The listing builds one solid part. Answer for the finished solid, in the listing's coordinates (mm). A direction names the side the tool comes from. Round coordinates to 2 decimals unless told otherwise and drop trailing zeros. Order: outer loops, then holes, each group sorted by start corner. A loop starts at its lowest first (then second) coordinate and runs counter-clockwise, first axis right, second up. Notation, with made-up numbers: (86.5, 51.25) - (138.5, 51.25) arc R13 cw to (138.5, 73.25) - close; hole circle Ø8 at (83.25, 27). An arc over 180 degrees is marked (long way). One line per item, written item: value. Start each with the question number.
1. Section A-A, the plane z = 5.75 is taken. Give the vertices of the cut face in (x, y), then the cut area to 3 significant figures.
2. Section D-D, the plane z = 9.75 is taken. Give the vertices of the cut face in (x, y), then the cut area to 3 significant figures.
3. Flat-ended cylindrical pins translate along their axes: P1, Ø6.5, axis at y = 41, z = 5, coming from the +X side; P2, Ø2, axis at x = 53, z = 3, coming from the +Y side; P3, Ø1.7, axis at x = 5.02, y = 31.5, coming from the +Z side; P4, Ø3.5, axis at x = 50.5, y = 46, coming from the -Z side. Find the tip coordinate at first contact, or state that the pin passes through.
4. For a pull along X with two mould halves and no side action, classify faces 1 (the flat face through (21, 36, 6)), 2 (the flat face through (0, 18, 6)), 3 (the flat face through (21.335, 18, 5)) as released by +X, released by -X, zero draft, split by the parting line, or undercut.
5. Section C-C, the plane y = 6.5 is taken. Give the vertices of the cut face in (x, z).
6. A tool of negligible diameter and unlimited length cuts with its end or side. For faces 4 (the flat face through (44, 21, 1)), 5 (the flat face through (43, 44, 7)), 6 (the flat face through (51, 44, 9)), 7 (the flat face through (33.7, 18, 5)), from which of +Z, -Z, +X, -X, +Y, -Y can it reach the whole face along a straight path? Write none if from no direction.
7. Straight lines are drawn through the part: line 1 (X direction, y = 21, z = 7); line 2 (X direction, y = 7, z = 10.75); line 3 (Z direction, x = 30, y = 21). For each, find the intervals that lie inside material, in ascending order.
8. Section B-B, the plane y = 39.3 is taken. Give the vertices of the cut face in (x, z).
Autodesk Inventor part; units mm, degrees
ref_plane "Work Plane2" through (38.0184, 32.2776, 9) normal (0, 0, 1) x (1, 0, 0)
ref_plane "YZ Plane" through (0, 0, 0) normal (1, 0, 0) x (0, 1, 0)
ref_plane "XZ Plane" through (0, 0, 0) normal (0, 1, 0) x (-1, 0, 0)
ref_plane "Work Plane1" through (22.0339, 196.5, 8) normal (0, 0, 1) x (1, 0, 0)
sketch "Sketch1" plane through (22.0339, 196.5, 8) normal (0, 0, 1) x (1, 0, 0)
  circle A0 centre (5.4838, -190) radius 1.4
  circle A1 centre (27.9838, -190) radius 1.4
  circle A2 centre (-17.0162, -190) radius 1.4
  line L0 (-22.0339, -196.5) -> (32.9661, -196.5)
  line L1 (32.9661, -196.5) -> (32.9661, -186.5)
  line L2 (-22.0339, -186.5) -> (32.9661, -186.5)
  line L3 (-22.0339, -196.5) -> (-22.0339, -186.5)
  circle A3 centre (27.9838, -165) radius 1.4
  circle A4 centre (-17.0162, -165) radius 1.4
  circle A5 centre (5.4838, -165) radius 1.4
  line L4 (32.9661, -160.5) -> (32.9661, -169.5)
  line L5 (-22.0339, -160.5) -> (32.9661, -160.5)
  line L6 (-22.0339, -160.5) -> (-22.0339, -169.5)
  line L7 (32.9661, -169.5) -> (-22.0339, -169.5)
  line L8 (32.9661, -196.5) -> (-22.0339, -196.5)
  line L9 (-22.0339, -196.5) -> (-22.0339, -160.5)
  line L10 (-22.0339, -160.5) -> (32.9661, -160.5)
  line L11 (32.9661, -160.5) -> (32.9661, -196.5)
extrude "Extrusion1" add sketch "Sketch1" along normal blind 4
sketch "Sketch2" plane through (22.0339, 196.5, 8) normal (0, 0, -1) x (-1, 0, 0)
  circle A0 centre (17.0162, -190) radius 1.4
  circle A1 centre (-27.9838, -190) radius 1.4
  circle A2 centre (-5.4838, -190) radius 1.4
  circle A3 centre (-5.4838, -165) radius 1.4
  circle A4 centre (17.0162, -165) radius 1.4
  circle A5 centre (-27.9838, -165) radius 1.4
  line L0 (-32.9661, -196.5) -> (-32.9661, -160.5)
  line L1 (22.0339, -196.5) -> (-32.9661, -196.5)
  line L2 (22.0339, -160.5) -> (22.0339, -196.5)
  line L3 (-32.9661, -160.5) -> (22.0339, -160.5)
  line L4 (22.0339, -196.5) -> (-32.9661, -196.5)
  line L5 (22.0339, -160.5) -> (0.6985, -160.5)
  line L6 (0.6985, -160.5) -> (0.6985, -196.5)
  line L7 (0.6985, -196.5) -> (22.0339, -196.5)
  line L8 (22.0339, -196.5) -> (22.0339, -160.5)
  line L9 (-32.9661, -196.5) -> (-32.9661, -160.5)
  line L10 (-32.9661, -160.5) -> (-11.6661, -160.5)
  line L11 (-11.6661, -160.5) -> (-11.6661, -196.5)
  line L12 (-11.6661, -196.5) -> (-32.9661, -196.5)
  line L13 (-32.9661, -196.5) -> (-32.9661, -160.5)
  line L14 (-11.4661, 0) -> (-11.4661, -200)
  line L15 (0.4985, 0) -> (0.4985, -200)
  dimension "d6" = 0.2
  dimension "d7" = 0.2
extrude "Extrusion2" add sketch "Sketch2" along normal blind 7 contours L0 L3 L11 L1 | L6 L3 L2 L1
sketch "Sketch3" plane through (22.0339, 196.5, 12) normal (0, 0, 1) x (1, 0, 0)
  circle A0 centre (-17.0162, -190) radius 1.4
  circle A1 centre (27.9838, -190) radius 1.4
  circle A2 centre (5.4838, -190) radius 1.4
  circle A3 centre (5.4838, -165) radius 1.4
  circle A4 centre (-17.0162, -165) radius 1.4
  circle A5 centre (27.9838, -165) radius 1.4
  line L0 (32.9661, -196.5) -> (32.9661, -160.5)
  line L1 (32.9661, -160.5) -> (-22.0339, -160.5)
  line L2 (-22.0339, -160.5) -> (-22.0339, -196.5)
  line L3 (-22.0339, -196.5) -> (32.9661, -196.5)
  circle A6 centre (28.987, -157.2) radius 1
  circle A7 centre (28.987, -157.2) radius 1
  circle A8 centre (50.837, -147.5) radius 1
  line L4 (53.837, -158.2) -> (53.837, -154.2581)
  line L5 (53.837, -154.2581) -> (61.5817, -154.2581)
  line L6 (61.5817, -154.2581) -> (61.5817, -153.1829)
  line L7 (61.5817, -153.1829) -> (53.837, -153.1829)
  line L8 (53.837, -153.1829) -> (53.837, -149.448)
  line L9 (53.837, -149.448) -> (61.5817, -149.448)
  line L10 (61.5817, -149.448) -> (61.5817, -148.769)
  line L11 (61.5817, -148.769) -> (53.837, -148.769)
  line L12 (53.837, -148.769) -> (53.837, -146.5)
  arc A9 (53.837, -146.5) -> (51.837, -144.5) centre (51.837, -146.5) ccw
  line L13 (51.837, -144.5) -> (46.3523, -144.5)
  line L14 (46.3523, -144.5) -> (18.7709, -139.6366)
  line L15 (18.7709, -139.6366) -> (16.0392, -139.155)
  line L16 (16.0392, -139.155) -> (15.987, -139.4512)
  line L17 (15.987, -139.4512) -> (44.6201, -144.5)
  line L18 (44.6201, -144.5) -> (27.987, -144.5)
  arc A10 (27.987, -144.5) -> (25.987, -146.5) centre (27.987, -146.5) ccw
  line L19 (25.987, -146.5) -> (25.987, -158.2)
  arc A11 (25.987, -158.2) -> (27.987, -160.2) centre (27.987, -158.2) ccw
  line L20 (27.987, -160.2) -> (33.9661, -160.2)
  line L21 (33.9661, -164.2178) -> (33.9661, -160.2)
  line L22 (42.5677, -164.2178) -> (33.9661, -164.2178)
  line L23 (42.5677, -164.2178) -> (42.5677, -163.1992)
  line L24 (42.5677, -163.1992) -> (35.1545, -163.1992)
  line L25 (35.1545, -160.2) -> (35.1545, -163.1992)
  line L26 (35.1545, -160.2) -> (51.837, -160.2)
  arc A12 (51.837, -160.2) -> (53.837, -158.2) centre (51.837, -158.2) ccw
  line L27 (32.9661, -160.5) -> (-22.0339, -160.5)
  line L28 (20.9661, -160.5) -> (32.9661, -160.5)
  line L29 (32.9661, -160.5) -> (32.9661, -144.5)
  line L30 (32.9661, -144.5) -> (20.9661, -144.5)
  line L31 (20.9661, -144.5) -> (20.9661, -160.5)
  point P0 (-22.0339, -196.5)
  dimension "d8" = 12
ref_plane "Work Plane2" through (38.0184, 32.2776, 9) normal (0, 0, 1) x (1, 0, 0)
extrude "Extrusion3" add sketch "Sketch3" against normal up to surface (3 mm away) contours L1 L31 L30 A10 L19 A11 L20 L29 | L20 A11 L19 A10 L18 L29
sketch "Sketch4" plane through (55, 52, 9) normal (0, 0, -1) x (-1, 0, 0)
  circle A0 centre (3.9791, -12.7) radius 1
  circle A1 centre (-17.8709, -3) radius 1
  line L0 (-20.8709, -13.7) -> (-20.8709, -9.7581)
  line L1 (-20.8709, -9.7581) -> (-28.6156, -9.7581)
  line L2 (-28.6156, -9.7581) -> (-28.6156, -8.6829)
  line L3 (-28.6156, -8.6829) -> (-20.8709, -8.6829)
  line L4 (-20.8709, -8.6829) -> (-20.8709, -4.948)
  line L5 (-20.8709, -4.948) -> (-28.6156, -4.948)
  line L6 (-28.6156, -4.948) -> (-28.6156, -4.269)
  line L7 (-28.6156, -4.269) -> (-20.8709, -4.269)
  line L8 (-20.8709, -4.269) -> (-20.8709, -2)
  arc A2 (-18.8709, 0) -> (-20.8709, -2) centre (-18.8709, -2) ccw
  line L9 (-18.8709, 0) -> (-13.3862, 0)
  line L10 (-13.3862, 0) -> (14.1952, 4.8634)
  line L11 (14.1952, 4.8634) -> (16.9269, 5.345)
  line L12 (16.9269, 5.345) -> (16.9791, 5.0488)
  line L13 (16.9791, 5.0488) -> (-11.654, 0)
  line L14 (-11.654, 0) -> (4.9791, 0)
  arc A3 (6.9791, -2) -> (4.9791, 0) centre (4.9791, -2) ccw
  line L15 (6.9791, -2) -> (6.9791, -13.7)
  arc A4 (4.9791, -15.7) -> (6.9791, -13.7) centre (4.9791, -13.7) ccw
  line L16 (4.9791, -15.7) -> (-1, -15.7)
  line L17 (-1, -19.7178) -> (-1, -15.7)
  line L18 (-9.6016, -19.7178) -> (-1, -19.7178)
  line L19 (-9.6016, -19.7178) -> (-9.6016, -18.6992)
  line L20 (-9.6016, -18.6992) -> (-2.1884, -18.6992)
  line L21 (-2.1884, -15.7) -> (-2.1884, -18.6992)
  line L22 (-2.1884, -15.7) -> (-18.8709, -15.7)
  arc A5 (-20.8709, -13.7) -> (-18.8709, -15.7) centre (-18.8709, -13.7) ccw
  line L23 (12, -16) -> (55, -16)
  circle A6 centre (3.9791, -12.7) radius 1
  circle A7 centre (49.9823, -45.5) radius 1.4
  circle A8 centre (4.9823, -45.5) radius 1.4
  circle A9 centre (27.4823, -45.5) radius 1.4
  circle A10 centre (27.4823, -20.5) radius 1.4
  circle A11 centre (49.9823, -20.5) radius 1.4
  circle A12 centre (4.9823, -20.5) radius 1.4
  line L24 (0, -52) -> (0, 0)
  line L25 (0, 0) -> (12, 0)
  line L26 (12, 0) -> (12, -16)
  line L27 (12, -16) -> (55, -16)
  line L28 (55, -16) -> (55, -52)
  line L29 (55, -52) -> (0, -52)
  line L30 (12, -16) -> (0, -16)
  line L31 (12, 0) -> (0, 0)
  line L32 (12, -16) -> (7.2, -16)
  line L33 (7.2, -16) -> (7.2, 0)
  line L34 (7.2, 0) -> (12, 0)
  line L35 (12, 0) -> (12, -16)
  point P0 (55, -52)
  dimension "d11" = 4.8
extrude "Extrusion4" add sketch "Sketch4" along normal up to surface (8 mm away) contours L33 L25 L26 L30
properties part number "04_Mount_Rail_Fastener"
Answer list:
1. outline: (0, 0) - (21.34, 0) - (21.34, 36) - (0, 36) - close; (33.7, 0) - (55, 0) - (55, 36) - (47.8, 36) - (47.8, 52) - (43, 52) - (43, 36) - (33.7, 36) - close; hole circle Ø2.8 at (5.02, 6.5); hole circle Ø2.8 at (5.02, 31.5); hole circle Ø2.8 at (50.02, 6.5); hole circle Ø2.8 at (50.02, 31.5)
1. area: 1,590 mm²
2. outline: (0, 0) - (55, 0) - (55, 52) - (43, 52) - (43, 36) - (0, 36) - close; hole circle Ø2.8 at (5.02, 6.5); hole circle Ø2.8 at (5.02, 31.5); hole circle Ø2.8 at (27.52, 6.5); hole circle Ø2.8 at (27.52, 31.5); hole circle Ø2.8 at (50.02, 6.5); hole circle Ø2.8 at (50.02, 31.5); hole circle Ø2 at (51.02, 39.3)
2. area: 2,130 mm²
3. P1: stops at x = 47.8
3. P2: stops at y = 36
3. P3: passes through
3. P4: stops at z = 9
4. face 1: zero draft
4. face 2: released by -X
4. face 3: undercut
5. outline: (0, 1) - (3.62, 1) - (3.62, 12) - (0, 12) - close; (6.42, 1) - (21.34, 1) - (21.34, 8) - (26.12, 8) - (26.12, 12) - (6.42, 12) - close; (28.92, 8) - (33.7, 8) - (33.7, 1) - (48.62, 1) - (48.62, 12) - (28.92, 12) - close; (51.42, 1) - (55, 1) - (55, 12) - (51.42, 12) - close
6. face 4: -Z, +X, -X, +Y, -Y
6. face 5: +Z, -Z, -X, +Y
6. face 6: -Z, +X, +Y
6. face 7: -Z, +Y, -Y
7. line 1: x = 0 to 21.34, 33.7 to 55
7. line 2: x = 0 to 3.71, 6.33 to 26.21, 28.83 to 48.71, 51.33 to 55
7. line 3: z = 8 to 12
8. outline: (43, 1) - (47.8, 1) - (47.8, 9) - (50.02, 9) - (50.02, 12) - (43, 12) - close; (52.02, 9) - (55, 9) - (55, 12) - (52.02, 12) - close
